Input: part model. Units: mm. Frame: model coordinates. A direction names the side the tool comes from. Round coordinates to 2 decimals unless told otherwise and drop trailing zeros. Write each loop counter-clockwise with the first axis right and the second up, starting at its lowest first coordinate (ties: lowest second). Pieces come first, ordered by that corner, then holes. Notation, with made-up numbers: (7.25, -19) -> (32.25, -19) arc R24 ccw to (32.25, 19) -> close; hole circle Ø10 at (15, -5). An arc over 180 degrees is marked (long way). Write item = value, one per line. Start each with the question number.
```python
from build123d import *
from OCP.BRepFilletAPI import BRepFilletAPI_MakeChamfer

# Parameters (mm, degrees)
SKETCH1_W           = 50
SKETCH1_H           = 60
BOSS_EXTRUDE1_DEPTH = 40
BOSS_EXTRUDE2_DEPTH = 60
SKETCH3_W           = 35
SKETCH3_H           = 45
CUT_EXTRUDE1_DEPTH  = 8
CUT_EXTRUDE1_DRAFT  = 25
SKETCH4_R           = 4
BOSS_EXTRUDE3_DEPTH = 5
SKETCH5_W           = 12
SKETCH5_H           = 35
BOSS_EXTRUDE4_DEPTH = 8
CHAMFER1_SIZE       = 3
CHAMFER1_SIZE2      = 10
CHAMFER2_SIZE       = 10
CHAMFER2_SIZE2      = 3


with BuildPart() as part:
    # Sketch1 → Boss-Extrude1 (new body)
    with BuildSketch(Plane(origin=(0, 0, 0), x_dir=(1, 0, 0), z_dir=(0, 1, 0))):
        Rectangle(SKETCH1_W, SKETCH1_H)
    extrude(amount=BOSS_EXTRUDE1_DEPTH)

    # Sketch2 → Boss-Extrude2 (add)
    with BuildSketch(Plane.XY.offset(30)):
        with BuildLine():
            Line((53.495378078, 29.369222598), (25, 40))
            Line((25, 40), (25, 0))
            Line((25, 0), (60, 0))
            Line((60, 0), (60, 20))
            ThreePointArc((60, 20), (58.214431836, 25.702903612), (53.495378078, 29.369222598))
        make_face()
    extrude(amount=-BOSS_EXTRUDE2_DEPTH)


with BuildPart() as cut_extrude1_tool:
    # Sketch3 → Cut-Extrude1 (with draft: the straight prism first)
    with BuildSketch(Plane(origin=(0, 40, 0), x_dir=(1, 0, 0), z_dir=(0, 1, 0))):
        Rectangle(SKETCH3_W, SKETCH3_H)
    extrude(amount=-CUT_EXTRUDE1_DEPTH)
    # Cut-Extrude1: the draft: its side faces are tilted about the plane it starts from
    cut_extrude1_sides = [cut_extrude1_tool.faces().sort_by_distance(p)[0] for p in [
        (0, 36, 22.5),
        (17.5, 36, 0),
        (0, 36, -22.5),
        (-17.5, 36, 0),
    ]]
    draft(cut_extrude1_sides, Plane(origin=(0, 40, 0), x_dir=(1, 0, 0), z_dir=(0, 1, 0)), CUT_EXTRUDE1_DRAFT)


with BuildPart() as part_1:
    add(part.part)

    # Cut-Extrude1: cut by cut_extrude1_tool
    add(cut_extrude1_tool.part, mode=Mode.SUBTRACT)

    # Sketch4 → Boss-Extrude3 (add)
    with BuildSketch(Plane.XY.offset(30)):
        with Locations(Location((50, 20, 0), (0, 0, 180))):
            Circle(SKETCH4_R)
    extrude(amount=BOSS_EXTRUDE3_DEPTH)

    # Sketch5 → Boss-Extrude4 (add)
    with BuildSketch(Plane.XY.offset(35)):
        with Locations((50, 20)):
            Rectangle(SKETCH5_W, SKETCH5_H)
    extrude(amount=BOSS_EXTRUDE4_DEPTH)

    # Chamfer1: one chamfer whose edges measure the first distance from different faces: ONE call of the kernel's chamfer builder (chamfer() names one face for all edges)
    chamfer1_edges_1 = [part_1.edges().sort_by_distance(p)[0] for p in [
        (56, 2.5, 39),
    ]]
    chamfer1_side_1 = [part_1.faces().sort_by_distance(p)[0] for p in [
        (50, 2.5, 39),
    ]]
    chamfer1_edges_2 = [part_1.edges().sort_by_distance(p)[0] for p in [
        (44, 37.5, 39),
    ]]
    chamfer1_side_2 = [part_1.faces().sort_by_distance(p)[0] for p in [
        (50, 37.5, 39),
    ]]
    chamfer1 = BRepFilletAPI_MakeChamfer(part_1.part.solid().wrapped)
    for e in chamfer1_edges_1:
        chamfer1.Add(CHAMFER1_SIZE, CHAMFER1_SIZE2, e.wrapped, chamfer1_side_1[0].wrapped)  # the first distance lies on this face
    for e in chamfer1_edges_2:
        chamfer1.Add(CHAMFER1_SIZE, CHAMFER1_SIZE2, e.wrapped, chamfer1_side_2[0].wrapped)  # the first distance lies on this face
    add(Compound.cast(chamfer1.Shape()), mode=Mode.REPLACE)

    # Chamfer2: one chamfer whose edges measure the first distance from different faces: ONE call of the kernel's chamfer builder (chamfer() names one face for all edges)
    chamfer2_edges_1 = [part_1.edges().sort_by_distance(p)[0] for p in [
        (56, 37.5, 39),
    ]]
    chamfer2_side_1 = [part_1.faces().sort_by_distance(p)[0] for p in [
        (56, 25, 39),
    ]]
    chamfer2_edges_2 = [part_1.edges().sort_by_distance(p)[0] for p in [
        (44, 2.5, 39),
    ]]
    chamfer2_side_2 = [part_1.faces().sort_by_distance(p)[0] for p in [
        (44, 15, 39),
    ]]
    chamfer2 = BRepFilletAPI_MakeChamfer(part_1.part.solid().wrapped)
    for e in chamfer2_edges_1:
        chamfer2.Add(CHAMFER2_SIZE, CHAMFER2_SIZE2, e.wrapped, chamfer2_side_1[0].wrapped)  # the first distance lies on this face
    for e in chamfer2_edges_2:
        chamfer2.Add(CHAMFER2_SIZE, CHAMFER2_SIZE2, e.wrapped, chamfer2_side_2[0].wrapped)  # the first distance lies on this face
    add(Compound.cast(chamfer2.Shape()), mode=Mode.REPLACE)


solid = part_1.part
```
1. Reachability of faces 1 (the flat face through (44, 20, 39)), 2 (the cylindrical face through (52.95, 17.3, 32.47)), 3 (the flat face through (54.52, 7.57, 38.94)) from +Z, -Z, +X, -X, +Y, -Y: full face, straight path, thin tool, end or side. Return the list, or none.
2. Pin query (flat end, axial travel): P1, Ø6.5, axis at y = 21.5, z = 37.5, coming from the -X side; P2, Ø3, axis at x = 49.5, z = 38, coming from the +Y side; P3, Ø6.5, axis at x = 49.5, z = 40.5, coming from the -Y side. Return the tip coordinate at first contact, or that it passes through.
3. Mould query, pull axis Z, two halves, no side actions, for faces 4 (the flat face through (-0.297, 36.056, 24.339)), 5 (the flat face through (50, 37.5, 39)), 6 (the flat face through (50, 20, 43)), 7 (the flat face through (17, 20, -30)). Classes: pulls with the +Z half, pulls with the -Z half, needs draft (parallel to the pull), parting line crosses it, or undercut.
4. Line query: line 1 along Z through (x, y) = (45.5, 24.5); line 2 along Z through (x, y) = (20.5, 37); line 3 along X through (y, z) = (28, 6). Output: solid intervals per line, ascending.
5. Section C-C (z = 10). Output: boundary loops of the cut face in (x, y).
6. Section B-B (x = 16.5). Output: boundary loops of the cut face in (y, z).
7. Section A-A (y = 11). Output: boundary loops of the cut face in (x, z).
8. Section D-D (z = 37). Output: boundary loops of the cut face in (x, y), then the cut area to 3 significant figures.
Check sheet entries:
q1.face_1 = +Z, -X, +Y, -Y
q1.face_2 = none
q1.face_3 = +Z, +X, -Y
q2.P1 = 44
q2.P2 = 37.5
q2.P3 = 2.5
q3.face_4 = undercut
q3.face_5 = needs draft
q3.face_6 = pulls with the +Z half
q3.face_7 = pulls with the -Z half
q4.line_1 = -30 to 30, 35 to 43
q4.line_2 = -30 to 30
q4.line_3 = -25 to 56
q5.outline = (-25, 0) -> (60, 0) -> (60, 20) arc R10 ccw to (53.5, 29.37) -> (25, 40) -> (17.5, 40) -> (21.23, 32) -> (-21.23, 32) -> (-17.5, 40) -> (-25, 40) -> close
q6.outline = (0, -30) -> (40, -30) -> (40, -22.5) -> (32, -26.23) -> (32, 26.23) -> (40, 22.5) -> (40, 30) -> (0, 30) -> close
q7.outline = (-25, -30) -> (60, -30) -> (60, 30) -> (-25, 30) -> close; (44.45, 35) -> (55.55, 35) -> (55.55, 43) -> (44.45, 43) -> close
q8.outline = (44, 12.5) -> (47, 2.5) -> (53, 2.5) -> (56, 12.5) -> (56, 27.5) -> (53, 37.5) -> (47, 37.5) -> (44, 27.5) -> close
q8.area = 360 mm2
